Geometry: final body of the model. Coordinates: model frame, mm. A direction names the side the tool comes from. Coordinates: 2 decimals unless noted, no trailing zeros. Loops run counter-clockwise (first coordinate to the right, second up) from the corner with the lowest first, then second, coordinate; pieces in that order, holes last. Notation, with made-up numbers: (65.5, 77.5) - (76.5, 77.5) arc R17 ccw to (76.5, 99.5) - close; hole circle Ø4 at (-24.75, 35.25). An arc over 180 degrees is marked (long way). Return JSON: item names as keys, results as strings.
from build123d import *

# Parameters (mm, degrees)
SKETCH1_R           = 40
BOSS_EXTRUDE1_DEPTH = 30
SKETCH2_R           = 30
BOSS_EXTRUDE2_DEPTH = 20
SKETCH3_R           = 20
BOSS_EXTRUDE3_DEPTH = 25
SKETCH4_R           = 12.5
BOSS_EXTRUDE4_DEPTH = 20
SKETCH5_OUTSIDE_W   = 111.546
SKETCH5_OUTSIDE_H   = 111.546
SKETCH5_OUTSIDE_W_2 = 20
SKETCH5_OUTSIDE_H_2 = 20
CUT_EXTRUDE2_DEPTH  = 15
CUT_EXTRUDE7_DEPTH  = 20
CUT_EXTRUDE8_START  = 50
CUT_EXTRUDE8_DEPTH  = 15
CUT_EXTRUDE9_DEPTH  = 20


with BuildPart() as part:
    # Sketch1 → Boss-Extrude1 (new body)
    with BuildSketch(Plane(origin=(0, 0, 0), x_dir=(1, 0, 0), z_dir=(0, 1, 0))):
        Circle(SKETCH1_R)
    extrude(amount=BOSS_EXTRUDE1_DEPTH)

    # Sketch2 → Boss-Extrude2 (add)
    with BuildSketch(Plane(origin=(0, 30, 0), x_dir=(1, 0, 0), z_dir=(0, 1, 0))):
        Circle(SKETCH2_R)
    extrude(amount=BOSS_EXTRUDE2_DEPTH)

    # Sketch3 → Boss-Extrude3 (add)
    with BuildSketch(Plane(origin=(0, 50, 0), x_dir=(1, 0, 0), z_dir=(0, 1, 0))):
        Circle(SKETCH3_R)
    extrude(amount=BOSS_EXTRUDE3_DEPTH)

    # Sketch4 → Boss-Extrude4 (add)
    with BuildSketch(Plane(origin=(0, 75, 0), x_dir=(1, 0, 0), z_dir=(0, 1, 0))):
        Circle(SKETCH4_R)
    extrude(amount=BOSS_EXTRUDE4_DEPTH)

    # Sketch5 outside → Cut-Extrude2 (cut)
    with BuildSketch(Plane(origin=(0, 95, 0), x_dir=(1, 0, 0), z_dir=(0, 1, 0))):
        Rectangle(SKETCH5_OUTSIDE_W, SKETCH5_OUTSIDE_H)
        Rectangle(SKETCH5_OUTSIDE_W_2, SKETCH5_OUTSIDE_H_2, mode=Mode.SUBTRACT)
    extrude(amount=-CUT_EXTRUDE2_DEPTH, mode=Mode.SUBTRACT)

    # Sketch6 → Cut-Extrude7 (cut)
    with BuildSketch(Plane(origin=(0, 75, 0), x_dir=(1, 0, 0), z_dir=(0, 1, 0))):
        Polygon((-5.77591504, 20.949618127), (-15, 15), (15, 15), (14.22408496, 20.949618127), align=None)
        Polygon((-15, -15), (-15, 15), (-20.949618127, 14.22408496), (-20.949618127, -5.77591504), align=None)
        Polygon((20.949618127, 5.77591504), (15, 15), (15, -15), (20.949618127, -14.22408496), align=None)
        Polygon((15, -15), (-15, -15), (-14.22408496, -20.949618127), (5.77591504, -20.949618127), align=None)
    extrude(amount=-CUT_EXTRUDE7_DEPTH, mode=Mode.SUBTRACT)

    # Sketch7 → Cut-Extrude8 (cut)
    with BuildSketch(Plane(origin=(0, 0, 0), x_dir=(1, 0, 0), z_dir=(0, 1, 0)).offset(CUT_EXTRUDE8_START)):
        with BuildLine():
            Line((-24.918588748, 25), (24.918588748, 25))
            ThreePointArc((24.918588748, 25), (0, 35.297819553), (-24.918588748, 25))
        make_face()
        with BuildLine():
            Line((25, 24.918588748), (25, -24.918588748))
            ThreePointArc((25, -24.918588748), (35.297819553, 0), (25, 24.918588748))
        make_face()
        with BuildLine():
            Line((24.918588748, -25), (-24.918588748, -25))
            ThreePointArc((-24.918588748, -25), (0, -35.297819553), (24.918588748, -25))
        make_face()
        with BuildLine():
            Line((-25, -24.918588748), (-25, 24.918588748))
            ThreePointArc((-25, 24.918588748), (-35.297819553, 0), (-25, -24.918588748))
        make_face()
    extrude(amount=-CUT_EXTRUDE8_DEPTH, mode=Mode.SUBTRACT)

    # Sketch8 → Cut-Extrude9 (cut)
    with BuildSketch(Plane(origin=(0, 30, 0), x_dir=(1, 0, 0), z_dir=(0, 1, 0))):
        with BuildLine():
            Line((-35, 35.707142143), (-35, 35))
            Line((-35, 35), (35, 35))
            Line((35, 35), (35, 35.707142143))
            ThreePointArc((35, 35.707142143), (0, 50), (-35, 35.707142143))
        make_face()
        with BuildLine():
            Line((-35, 35), (-35.707142143, 35))
            ThreePointArc((-35.707142143, 35), (-50, 0), (-35.707142143, -35))
            Line((-35.707142143, -35), (-35, -35))
            Line((-35, -35), (-35, 35))
        make_face()
        with BuildLine():
            Line((35.707142143, 35), (35, 35))
            Line((35, 35), (35, -35))
            Line((35, -35), (35.707142143, -35))
            ThreePointArc((35.707142143, -35), (50, 0), (35.707142143, 35))
        make_face()
        with BuildLine():
            Line((35, -35), (-35, -35))
            Line((-35, -35), (-35, -35.707142143))
            ThreePointArc((-35, -35.707142143), (0, -50), (35, -35.707142143))
            Line((35, -35.707142143), (35, -35))
        make_face()
    extrude(amount=-CUT_EXTRUDE9_DEPTH, mode=Mode.SUBTRACT)


solid = part.part
Item 1: Reachability of faces 1 (the face through (0, 20, -35)), 2 (the face through (17, 55, 0)), 3 (the face through (-12.488, 78.193, -0.55)), 4 (the face through (-11, 80, 0)) from +Z, -Z, +X, -X, +Y, -Y: full face, straight path, thin tool, end or side. Return the list, or none.
Worked out:
{"face 1": "-Z, +X, -X, +Y", "face 2": "+Z, -Z, +X, +Y", "face 3": "+Y", "face 4": "+Z, -Z, -X, +Y"}
Item 2: First-contact query: pin 1 Ø6 at (y, z) = (24.5, 2) entering from -X; pin 2 Ø1.5 at (x, z) = (8, -37.5) entering from +Y; pin 3 Ø3 at (y, z) = (53, 2) entering from +X. Flat tips, straight axial feed; report the tip coordinate or a pass-through.
Worked out:
{"pin 1": "x = -35", "pin 2": "y = 10", "pin 3": "x = 19.99"}
Item 3: Ray query, probe 1 along Y at (x, z) = (36, 9); probe 2 along Z at (x, y) = (9.5, 57); probe 3 along Y at (x, z) = (-22, 3.5). Return the intervals inside material, ascending. Write a range as from..to.
Worked out:
{"probe 1": "0..10", "probe 2": "-15..15", "probe 3": "0..50"}
Item 4: Section query A-A, the plane y = 15.5. Return loops of the section in (x, z).
Worked out:
{"outline": "(-35, -19.36) arc R40 ccw to (-19.36, -35) - (19.36, -35) arc R40 ccw to (35, -19.36) - (35, 19.36) arc R40 ccw to (19.36, 35) - (-19.36, 35) arc R40 ccw to (-35, 19.36) - close"}
Item 5: Section query D-D, the plane y = 45. Return loops of the section in (x, z).
Worked out:
{"outline": "(-25, -16.58) arc R30 ccw to (-16.58, -25) - (16.58, -25) arc R30 ccw to (25, -16.58) - (25, 16.58) arc R30 ccw to (16.58, 25) - (-16.58, 25) arc R30 ccw to (-25, 16.58) - close"}
